Autodesk Fusion 360 part; units mm, degrees
sketch "Box base" plane through (0, 0, 0) normal (0, 1, 0) x (1, 0, 0)
  line L0 (55, -40) -> (-55, -40)
  line L1 (-55, -40) -> (-55, 40)
  line L2 (-55, 40) -> (55, 40)
  line L3 (55, 40) -> (55, -40)
  line L4 (55, -40) -> (-55, 40) construction
  line L5 (-55, -40) -> (55, 40) construction
  dimension "d3" = 110
  dimension "d4" = 80
extrude "Extrude2" add sketch "Box base" along normal blind 35
sketch "Center box" plane through (0, 35, 0) normal (0, 1, 0) x (-1, 0, 0)
  line L0 (-55, -40) -> (55, -40)
  line L1 (55, -40) -> (55, 40)
  line L2 (55, 40) -> (-55, 40)
  line L3 (-55, 40) -> (-55, -40)
  line L4 (-50, 35) -> (50, 35)
  line L5 (50, 35) -> (50, -35)
  line L6 (50, -35) -> (-50, -35)
  line L7 (-50, -35) -> (-50, 35)
  line L8 (-50, 35) -> (50, -35) construction
  line L9 (50, 35) -> (-50, -35) construction
  dimension "d9" = 100
  dimension "d10" = 70
extrude "Extrude3" cut sketch "Center box" against normal blind 30 contours L4 L5 L6 L7
sketch "open one end" plane through (0, 0, 40) normal (0, 0, 1) x (1, 0, 0)
  line L0 (-55, 0) -> (55, 0)
  line L1 (55, 0) -> (55, 35)
  line L2 (55, 35) -> (-55, 35)
  line L3 (-55, 35) -> (-55, 0)
  line L4 (-55, 35) -> (55, 35)
  line L5 (55, 35) -> (55, 0)
  line L6 (55, 0) -> (-55, 0)
  line L7 (-55, 0) -> (-55, 35)
extrude "Extrude4" cut sketch "open one end" against normal blind 5
sketch "line marker for slit" plane through (0, 0, 35) normal (0, 0, 1) x (1, 0, 0)
  line L0 (-50, 5) -> (-50, 35)
  line L1 (-50, 35) -> (-55, 35)
  line L2 (-55, 35) -> (-55, 0)
  line L3 (-55, 0) -> (55, 0)
  line L4 (55, 0) -> (55, 35)
  line L5 (55, 35) -> (50, 35)
  line L6 (50, 35) -> (50, 5)
  line L7 (-50, 5) -> (-50, 29) construction
  line L8 (-50, 29) -> (-55, 29) construction
  line L9 (-55, 0) -> (-55, 35)
  line L10 (50, 5) -> (-50, 5)
  dimension "d21" = 24
sketch "Slit for diffuser" plane through (-55, 0, 0) normal (-1, 0, 0) x (0, 0, 1)
  line L0 (35, 0) -> (35, 35)
  line L1 (35, 35) -> (-40, 35)
  line L2 (-40, 35) -> (-40, 0)
  line L3 (-40, 0) -> (35, 0)
  line L4 (-40, 29) -> (35, 29) construction
  line L5 (-37.5, 30) -> (32.5, 30)
  line L6 (32.5, 30) -> (32.5, 29)
  line L7 (32.5, 29) -> (-37.5, 29)
  line L8 (-37.5, 29) -> (-37.5, 30)
  dimension "d22" = 70
  dimension "d23" = 1
extrude "Extrude6" cut sketch "Slit for diffuser" against normal up to surface (110 mm away) contours L5 L6 L7 L8
sketch "Sketch8" plane through (0, 35, 0) normal (0, 1, 0) x (-1, 0, 0)
  line L0 (4.5, -32.5) -> (-4.5, -32.5)
  line L1 (-4.5, -32.5) -> (-4.5, 32.5)
  line L2 (-4.5, 32.5) -> (4.5, 32.5)
  line L3 (4.5, 32.5) -> (4.5, -32.5)
  line L4 (4.5, -32.5) -> (-4.5, 32.5) construction
  line L5 (-4.5, -32.5) -> (4.5, 32.5) construction
  dimension "d28" = 9
  dimension "d29" = 65
extrude "Extrude7" cut sketch "Sketch8" against normal blind 31
pattern_linear "R-Pattern1" count 9 spacing 11 along (-1, 0, 0) both ways of "Extrude7"
sketch "nut holder" plane through (0, 0, 35) normal (0, 0, 1) x (1, 0, 0)
  line L0 (55, 10) -> (65, 10)
  line L1 (65, 10) -> (65, 0)
  line L2 (65, 0) -> (55, 0)
  line L3 (55, 0) -> (55, 10)
  circle A0 centre (60, 5) radius 2
  line L4 (60, 10) -> (60, 0) construction
  line L5 (65, 5) -> (55, 5) construction
  dimension "d36" = 10
  dimension "d37" = 10
  dimension "d43" = 4
extrude "Extrude8" add sketch "nut holder" against normal blind 4 contours L0 L1 L2 L3 | A0
extrude "Extrude9" cut sketch "nut holder" against normal blind 4 contours A0
fillet "Fillet1" radius 2 2 edges at (55, 10, 33) (55, 5, 31)
mirror "Mirror2" about plane through (0, 0, 0) normal (1, 0, 0) of "Extrude8", "Extrude9"
fillet "Fillet3" radius 2 2 edges at (-55, 10, 33) (-55, 5, 31)
fillet "Fillet4" radius 1 3 edges at (0, 35, -40) (-55, 35, -2.5) (55, 35, -2.5)
Verification items for the finished model (mm, model axes). A direction names the side the tool comes from. Coordinates: 2 decimals unless noted, no trailing zeros. Write each loop counter-clockwise with the first axis right and the second up, starting at its lowest first coordinate (ties: lowest second). Pieces come first, ordered by that corner, then holes. Notation, with made-up numbers: M 10,-0.5 L 28,-0.5 A8 ccw 28,10.5 Z; hole C -24,47 d6. An arc over 180 degrees is marked long. One line per item, written item: value.
Item 1: Section check A-A, the plane x = 60. Record the boundary of the cut face in (y, z), plus the area to 3 significant figures.
Check sheet entries:
outline: M 0,31 L 3,31 L 3,35 L 0,35 Z; M 7,31 L 10,31 L 10,35 L 7,35 Z
area: 24.0 mm^2
Item 2: Scan lines: line 1 along X through (y, z) = (12, -21.5); line 2 along Y through (x, z) = (60, 33.2); line 3 along Z through (x, y) = (-16.5, 18). Record each from-to range of solid material in increasing order.
Check sheet entries:
line 1: x = -55 to -50, 50 to 55
line 2: y = 0 to 3, 7 to 10
line 3: z = -40 to -35
Item 3: Mould release check, pull along Z, two halves, no side actions. Record for faces 1 (the flat face through (0, 3, 35)), 2 (the flat face through (-22, 4, 0)), 3 (the flat face through (-55, 17, -2)): pulls with the +Z half, pulls with the -Z half, needs draft (parallel to the pull), parting line crosses it, or undercut.
Check sheet entries:
face 1: pulls with the +Z half
face 2: undercut
face 3: needs draft
Item 4: Section check B-B, the plane x = 32. Record the boundary of the cut face in (y, z), plus the area to 3 significant figures.
Check sheet entries:
outline: M 0,-40 L 34,-40 A1 ccw 35,-39 L 35,-35 L 30,-35 L 30,-37.5 L 29,-37.5 L 29,-35 L 5,-35 L 5,-32.5 L 4,-32.5 L 4,32.5 L 5,32.5 L 5,35 L 0,35 Z
area: 457 mm^2
Item 5: Gauge pin test, flat ends, axial feed: pin 1 Ø4.5 at (x, z) = (-43.5, 11.5) entering from +Y; pin 2 Ø1.5 at (y, z) = (3.5, 9.5) entering from -X; pin 3 Ø0.5 at (y, z) = (4.5, -6) entering from +X. Record the tip position at first contact, or that the pin passes through.
Check sheet entries:
pin 1: stops at y = 4
pin 2: stops at x = -55
pin 3: stops at x = 55
Item 6: Access from +Z, -Z, +X, -X, +Y, -Y to the whole of each face (thin tool, end or side, straight path). Record for faces 4 (the flat face through (-11, 4, 0)), 5 (the flat face through (0, 30, -36)), 6 (the flat face through (61, 10, 33)).
Check sheet entries:
face 4: +Y
face 5: +X, -X
face 6: +Z, -Z, +X, +Y
Item 7: Section check C-C, the plane z = 15. State how many separate pieces and enclosed holes the cut face has, plus the area to 3 significant figures.
Check sheet entries:
separate pieces: 3
enclosed holes: 0
area: 759 mm^2
